from build123d import *

# Parameters (mm, degrees)
F1_DEPTH  = 100
F2_W      = 5
F2_H      = 10
F3_DEPTH  = 5
F4_R      = 0.875
F5_DEPTH  = 25
F6_R      = 0.4
F8_DEPTH  = 3.5
F9_DEPTH  = 11.001
F10_SIZE  = 0.5
F11_W     = 10
F11_H     = 5
F12_DEPTH = 25
F13_SIZE  = 0.4


with BuildPart() as f1:
    # F0 (on Front) → F1 (new body)
    with BuildSketch(Plane.XZ):
        Polygon((2.5, -2.5), (5, -2.5), (5, 2.5), (10, 2.5), (10, 4.5), (6, 4.5), (10, 8.5), (6, 8.5), (-6, 8.5), (-10, 8.5), (-6, 4.5), (-10, 4.5), (-10, 2.5), (-5, 2.5), (-5, -2.5), (-2.5, -2.5), (-2.5, 2.5), (2.5, 2.5), align=None)
    extrude(amount=F1_DEPTH)

    # F2 (on face) → F3 (join)
    with BuildSketch(Plane(origin=(0, 0, 2.5), x_dir=(1, 0, 0), z_dir=(0, 0, -1))):
        with Locations((0, 95)):
            Rectangle(F2_W, F2_H)
        Polygon((-2.5, 50), (-2.5, 45), (2.5, 45), (2.5, 50), (2.5, 55), (-2.5, 55), align=None)
        with Locations((0, 5)):
            Rectangle(F2_W, F2_H)
    extrude(amount=F3_DEPTH)

    # F4 (on face) → F5 (cut)
    with BuildSketch(Plane.YZ.offset(5)):
        with Locations((-85, 0)):
            Circle(F4_R)
        with Locations((-40, 0)):
            Circle(F4_R)
    extrude(amount=-F5_DEPTH, mode=Mode.SUBTRACT)

    # F6
    f6_edges = [f1.edges().sort_by_distance(p)[0] for p in [
        (10, -50, 4.5),
        (-10, -50, 4.5),
        (-6, -50, 4.5),
        (6, -50, 4.5),
        (10, -50, 8.5),
        (-10, -50, 8.5),
    ]]
    fillet(f6_edges, radius=F6_R)

    # F7 (on face) → F8 (cut)
    with BuildSketch(Plane.XY.offset(8.5)):
        with BuildLine():
            ThreePointArc((0, -92.2), (-2.8, -95), (0, -97.8))
            Line((0, -97.8), (0, -96.5))
            ThreePointArc((0, -96.5), (-1.5, -95), (0, -93.5))
            Line((0, -93.5), (0, -92.2))
        make_face()
        with BuildLine():
            ThreePointArc((0, -2.2), (-2.8, -5), (0, -7.8))
            Line((0, -7.8), (0, -6.5))
            ThreePointArc((0, -6.5), (-1.5, -5), (0, -3.5))
            Line((0, -3.5), (0, -2.2))
        make_face()
        with BuildLine():
            Line((0, -6.5), (0, -7.8))
            ThreePointArc((0, -7.8), (1.9798989873, -6.9798989873), (2.8, -5))
            ThreePointArc((2.8, -5), (1.9798989873, -3.0201010127), (0, -2.2))
            Line((0, -2.2), (0, -3.5))
            ThreePointArc((0, -3.5), (1.0606601718, -3.9393398282), (1.5, -5))
            ThreePointArc((1.5, -5), (1.0606601718, -6.0606601718), (0, -6.5))
        make_face()
        with BuildLine():
            ThreePointArc((0, -47.2), (-2.8, -50), (0, -52.8))
            Line((0, -52.8), (0, -51.5))
            ThreePointArc((0, -51.5), (-1.5, -50), (0, -48.5))
            Line((0, -48.5), (0, -47.2))
        make_face()
        with BuildLine():
            Line((0, -51.5), (0, -52.8))
            ThreePointArc((0, -52.8), (1.9798989873, -51.9798989873), (2.8, -50))
            ThreePointArc((2.8, -50), (1.9798989873, -48.0201010127), (0, -47.2))
            Line((0, -47.2), (0, -48.5))
            ThreePointArc((0, -48.5), (1.0606601718, -48.9393398282), (1.5, -50))
            ThreePointArc((1.5, -50), (1.0606601718, -51.0606601718), (0, -51.5))
        make_face()
        with BuildLine():
            Line((0, -96.5), (0, -97.8))
            ThreePointArc((0, -97.8), (1.9798989873, -96.9798989873), (2.8, -95))
            ThreePointArc((2.8, -95), (1.9798989873, -93.0201010127), (0, -92.2))
            Line((0, -92.2), (0, -93.5))
            ThreePointArc((0, -93.5), (1.0606601718, -93.9393398282), (1.5, -95))
            ThreePointArc((1.5, -95), (1.0606601718, -96.0606601718), (0, -96.5))
        make_face()
    extrude(amount=-F8_DEPTH, mode=Mode.SUBTRACT)

    # F9 (cut, through all): faces of the model
    f9_faces = [f1.faces().sort_by_distance(p)[0] for p in [
        (0, -5, 8.5),
        (0, -50, 8.5),
        (0, -95, 8.5),
    ]]
    extrude(f9_faces, amount=-F9_DEPTH, mode=Mode.SUBTRACT)

    # F10
    f10_edges = [f1.edges().sort_by_distance(p)[0] for p in [
        (0, -2.2, 8.5),
        (0, -47.2, 8.5),
        (0, -92.2, 8.5),
        (0, -6.5, 5),
        (0, -51.5, 5),
        (0, -96.5, 5),
        (0, -96.5, -2.5),
        (0, -51.5, -2.5),
        (0, -6.5, -2.5),
    ]]
    chamfer(f10_edges, length=F10_SIZE)

    # F11 (on face) → F12 (cut)
    with BuildSketch(Plane(origin=(-5, 0, 0), x_dir=(0, -1, 0), z_dir=(-1, 0, 0))):
        with Locations((5, 0)):
            Rectangle(F11_W, F11_H)
        with Locations((50, 0)):
            Rectangle(F11_W, F11_H)
        with Locations((95, 0)):
            Rectangle(F11_W, F11_H)
    extrude(amount=-F12_DEPTH, mode=Mode.SUBTRACT)

    # F13
    f13_edges = [f1.edges().sort_by_distance(p)[0] for p in [
        (5, -72.5, -2.5),
        (3.75, -90, -2.5),
        (2.5, -72.5, -2.5),
        (3.75, -55, -2.5),
        (-3.75, -55, -2.5),
        (-2.5, -72.5, -2.5),
        (-3.75, -90, -2.5),
        (-5, -72.5, -2.5),
        (-3.75, -10, -2.5),
        (-2.5, -27.5, -2.5),
        (-3.75, -45, -2.5),
        (-5, -27.5, -2.5),
        (5, -27.5, -2.5),
        (3.75, -45, -2.5),
        (2.5, -27.5, -2.5),
        (3.75, -10, -2.5),
        (2.5, -90, 0),
        (5, -90, 0),
        (3.75, -90, 2.5),
        (-5, -90, 0),
        (-2.5, -90, 0),
        (-3.75, -90, 2.5),
        (2.5, -45, 0),
        (5, -45, 0),
        (3.75, -45, 2.5),
        (-5, -45, 0),
        (-2.5, -45, 0),
        (-3.75, -45, 2.5),
        (2.5, -55, 0),
        (3.75, -55, 2.5),
        (5, -55, 0),
        (-5, -55, 0),
        (-3.75, -55, 2.5),
        (-2.5, -55, 0),
        (-5, -10, 0),
        (-3.75, -10, 2.5),
        (-2.5, -10, 0),
        (2.5, -10, 0),
        (3.75, -10, 2.5),
        (5, -10, 0),
        (5, -27.5, 2.5),
        (2.5, -27.5, 2.5),
        (-2.5, -27.5, 2.5),
        (-5, -27.5, 2.5),
        (5, -72.5, 2.5),
        (2.5, -72.5, 2.5),
        (-2.5, -72.5, 2.5),
        (-5, -72.5, 2.5),
    ]]
    chamfer(f13_edges, length=F13_SIZE)


solid = f1.part
Verification items for the finished model (mm, model axes). A direction names the side the tool comes from. Give positions to 0.01 mm unless a question says otherwise; leave off trailing zeros. Order: outer loops, then holes, each group sorted by start corner. A loop starts at its lowest first (then second) coordinate and runs counter-clockwise, first axis right, second up. Notation, with made-up numbers: M 54,52 L 100,52 A30 ccw 100,91 Z; hole C 30,25.25 d3. An arc over 180 degrees is marked long. Answer as a JSON object with one key per item and string values. Group by question number.
1) Access from +Z, -Z, +X, -X, +Y, -Y to the whole of each face (thin tool, end or side, straight path). Record for faces 4 (the face through (2.5, -72, 0)), 5 (the face through (-8, -49, 4.5)), 6 (the face through (4, -10, 0)), 7 (the face through (-5, -72, 0)), 8 (the face through (-2, -4, 5)).
2) Cross-section at A-A (z = 6.75). Enter the section's corners in (x, y), then the cut area to 3 significant figures.
3) Scan lines: line 1 along Y through (x, z) = (0, 5.5); line 2 along X through (y, z) = (-66.5, 1.5); line 3 along Z through (x, y) = (-4.2, -40) (3 decimals). Record each from-to range of solid material in increasing order. Write a range as [from, to].
4) Cross-section at C-C (y = -40). Give the number of separate pieces and of enclosed holes in the cut face, then the cut area to 3 significant figures.
5) Mould release check, pull along Y, two halves, no side actions. Record for faces 1 (the face through (0, -100, 6)), 2 (the face through (-4, -45, 0)), 3 (the face through (-2.5, -72, 0)): released by +Y, released by -Y, zero draft, split by the parting line, or undercut.
6) Depth check by flat-ended pin: pin 1 Ø2.5 at (y, z) = (-40, 0) entering from -X; pin 2 Ø0.9 at (x, z) = (3.5, -0.5) entering from -Y; pin 3 Ø1.9 at (x, z) = (-3.5, 0.5) entering from +Y. Enter the tip coordinate at first touch or a pass-through.
Result sheet:
{
 "1": {"face 4": "-Z, +Y, -Y", "face 5": "-X, +Y, -Y", "face 6": "-Z, +X, -X, +Y", "face 7": "-Z, -X, +Y, -Y", "face 8": "+Z"},
 "2": {"outline": "M -8.25,-100 L 8.25,-100 L 8.25,0 L -8.25,0 Z; hole C 0,-95 d5.6; hole C 0,-50 d5.6; hole C 0,-5 d5.6", "area": "1,580 mm2"},
 "3": {"line 1": "y = [-100, -97.8], [-92.2, -52.8], [-47.2, -7.8], [-2.2, 0]", "line 2": "x = [-5, -2.5], [2.5, 5]", "line 3": "z = [-2.5, -0.875], [0.875, 8.5]"},
 "4": {"separate pieces": "3", "enclosed holes": "0", "area": "120 mm2"},
 "5": {"face 1": "released by -Y", "face 2": "undercut", "face 3": "zero draft"},
 "6": {"pin 1": "stops at x = -5", "pin 2": "stops at y = -90", "pin 3": "stops at y = -10"}
}
